The model under review builds one solid part; all positions refer to its coordinate system, in mm. Round coordinates to 2 decimals unless told otherwise and drop trailing zeros. Write each loop counter-clockwise with the first axis right and the second up, starting at its lowest first coordinate (ties: lowest second). Pieces come first, ordered by that corner, then holes. Notation, with made-up numbers: (-7.75, 41.5) -> (33.25, 41.5) arc R19 ccw to (33.25, 67.5) -> close; hole circle Ø9 at (88, 28). An arc over 180 degrees is marked (long way). Answer as a JSON object with one key per item and string values. Group by question number.
1) To check wall thickness, follow probe 1 along Y at (x, z) = (4.05, -195); probe 2 along Z at (x, y) = (4.25, 275.5); probe 3 along Z at (x, y) = (2.5, 101). State the ranges of each line that lie inside material, in increasing order. Write a range as [from, to].
2) Mouldability with a two-part tool opening along Z and no side actions: class faces 1 (the flat face through (6, 188, -104)), 2 (the cylindrical face through (3, 352.6, -191.8)) as pulls with the +Z half, pulls with the -Z half, needs draft (parallel to the pull), parting line crosses it, or undercut.
3) We need section A-A, the plane y = 119. Write out the cut boundary in (x, z).
4) We need section C-C, the plane x = 2.7. Count the separate pieces of the cut face and the enclosed holes in it, then the cut area to 3 significant figures.
5) We need section D-D, the plane z = -147.5. Write out the cut boundary in (x, y).
6) We need section B-B, the plane z = -195. Write out the cut boundary in (x, y), then the cut area to 3 significant figures.
from build123d import *

# Parameters (mm, degrees)
SKETCH1_W           = 210
SKETCH1_H           = 370
BOSS_EXTRUDE1_DEPTH = 6
SKETCH2_W           = 50
SKETCH2_H           = 65
SKETCH2_W_2         = 19
SKETCH2_H_2         = 29
CUT_EXTRUDE1_DEPTH  = 10
SKETCH3_R           = 2
CUT_EXTRUDE2_DEPTH  = 10
SKETCH4_R           = 8
CUT_EXTRUDE3_DEPTH  = 10
SKETCH5_R           = 4
CUT_EXTRUDE4_DEPTH  = 12


with BuildPart() as part:
    # Sketch1 → Boss-Extrude1 (new body)
    with BuildSketch(Plane(origin=(0, 0, 0), x_dir=(0, 0, -1), z_dir=(1, 0, 0))):
        with Locations((105, 185)):
            Rectangle(SKETCH1_W, SKETCH1_H)
    extrude(amount=BOSS_EXTRUDE1_DEPTH)

    # Sketch2 → Cut-Extrude1 (cut)
    with BuildSketch(Plane.ZY):
        with Locations((-91.955439439, 96.451615806)):
            Rectangle(SKETCH2_W, SKETCH2_H)
        with Locations((-147.762028201, 286.067321943)):
            Rectangle(SKETCH2_W_2, SKETCH2_H_2)
        with Locations((-65.37786445, 286.067321943)):
            Rectangle(SKETCH2_W_2, SKETCH2_H_2)
    extrude(amount=-CUT_EXTRUDE1_DEPTH, mode=Mode.SUBTRACT)

    # Sketch3 → Cut-Extrude2 (cut)
    with BuildSketch(Plane.ZY):
        with Locations((-91.955439439, 133.951615806)):
            Circle(SKETCH3_R)
        with Locations((-91.955439439, 58.951615806)):
            Circle(SKETCH3_R)
    extrude(amount=-CUT_EXTRUDE2_DEPTH, mode=Mode.SUBTRACT)

    # Sketch4 → Cut-Extrude3 (cut)
    with BuildSketch(Plane(origin=(6, 0, 0), x_dir=(0, 0, -1), z_dir=(1, 0, 0))):
        with Locations((146.241614862, 335.160418709)):
            Circle(SKETCH4_R)
        with Locations((64.956823424, 335.160418709)):
            Circle(SKETCH4_R)
    extrude(amount=-CUT_EXTRUDE3_DEPTH, mode=Mode.SUBTRACT)

    # Sketch5 → Cut-Extrude4 (cut)
    with BuildSketch(Plane(origin=(6, 0, 0), x_dir=(0, 0, -1), z_dir=(1, 0, 0))):
        with Locations((15.00004659, 15.105743091)):
            Circle(SKETCH5_R)
        with Locations((15.00009318, 355.052871545)):
            Circle(SKETCH5_R)
        with Locations((195.00004659, 355)):
            Circle(SKETCH5_R)
        with Locations((195, 15.017639421)):
            Circle(SKETCH5_R)
    extrude(amount=-CUT_EXTRUDE4_DEPTH, mode=Mode.SUBTRACT)


solid = part.part
Here are the results:
{
 "1": {"probe 1": "y = [0, 11.02], [19.02, 351], [359, 370]", "probe 2": "z = [-210, -157.26], [-138.26, -74.88], [-55.88, 0]", "probe 3": "z = [-210, -116.96], [-66.96, 0]"},
 "2": {"face 1": "needs draft", "face 2": "undercut"},
 "3": {"outline": "(0, -210) -> (6, -210) -> (6, -116.96) -> (0, -116.96) -> close; (0, -66.96) -> (6, -66.96) -> (6, 0) -> (0, 0) -> close"},
 "4": {"separate pieces": "1", "enclosed holes": "11", "area": "72,700 mm^2"},
 "5": {"outline": "(0, 0) -> (6, 0) -> (6, 271.57) -> (0, 271.57) -> close; (0, 300.57) -> (6, 300.57) -> (6, 327.26) -> (0, 327.26) -> close; (0, 343.06) -> (6, 343.06) -> (6, 370) -> (0, 370) -> close"},
 "6": {"outline": "(0, 0) -> (6, 0) -> (6, 11.02) -> (0, 11.02) -> close; (0, 19.02) -> (6, 19.02) -> (6, 351) -> (0, 351) -> close; (0, 359) -> (6, 359) -> (6, 370) -> (0, 370) -> close", "area": "2,120 mm^2"}
}
